Verification items for the finished model (mm, model axes). A direction names the side the tool comes from. Round coordinates to 2 decimals unless told otherwise and drop trailing zeros. Order: outer loops, then holes, each group sorted by start corner. A loop starts at its lowest first (then second) coordinate and runs counter-clockwise, first axis right, second up. Notation, with made-up numbers: (10, 69.5) -> (49, 69.5) arc R17 cw to (49, 96.5) -> close; hole circle Ø1 at (-19, -35). An arc over 180 degrees is marked (long way). Return JSON: item names as keys, results as strings. Group by question number.
Item 1: Draft check along Z on faces 4 (the flat face through (19, 63, 1)), 5 (the flat face through (10, 26, 7)), 6 (the flat face through (10.14, 18.43, 19.94)). Enter one of: pulls with the +Z half, pulls with the -Z half, needs draft (parallel to the pull), parting line crosses it, or undercut.
Item 2: Sectioned sample at B-B on x = 55. Record the cut outline in (y, z) (3 decimals), plus the area to 3 significant figures.
Item 3: Depth check by flat-ended pin: pin 1 Ø1.6 at (x, y) = (10.5, 8.5) entering from -Z; pin 2 Ø4.5 at (x, y) = (55, 53) entering from +Z; pin 3 Ø12 at (x, z) = (57, -40) entering from -Y; pin 4 Ø3 at (x, y) = (41.5, 45.5) entering from -Z. Enter the tip coordinate at first touch or a pass-through.
Item 4: Scan lines: probe 1 along Y at (x, z) = (13, -5.5); probe 2 along Y at (x, z) = (55, 46); probe 3 along Z at (x, y) = (26.5, 50) (3 decimals). Record each from-to range of solid material in increasing order. Write a range as from..to.
Item 5: Sectioned sample at C-C on z = -32. Record the cut outline in (x, y), plus the area to 3 significant figures.
Item 6: Sectioned sample at A-A on y = 53. Record the cut outline in (x, z) (3 decimals), plus the area to 3 significant figures.
Item 7: Access from +Z, -Z, +X, -X, +Y, -Y to the whole of each face (thin tool, end or side, straight path). Record for faces 1 (the flat face through (35, 53, 34.545)), 2 (the flat face through (45, 43, 42)), 3 (the flat face through (10, 6, -7)).
Item 8: Sectioned sample at D-D on y = 14.5. Record the cut outline in (x, z).
```python
from build123d import *

# Parameters (mm, degrees)
BOSS_EXTRUDE1_DEPTH = 20
CUT_EXTRUDE1_DEPTH  = 20
SKETCH4_W           = 15
SKETCH4_H           = 20
BOSS_EXTRUDE2_DEPTH = 50
SKETCH5_R           = 2.5
CUT_EXTRUDE2_DEPTH  = 137.703431193
SKETCH6_W           = 8
SKETCH6_H           = 15
CUT_EXTRUDE3_DEPTH  = 95.465374741
CUT_EXTRUDE4_DEPTH  = 95.465374741


with BuildPart() as part:
    # Sketch1 → Boss-Extrude1 (new body)
    with BuildSketch(Plane(origin=(0, 0, 0), x_dir=(0, 0, -1), z_dir=(1, 0, 0))):
        Polygon((15, 0), (-15, 0), (-49.545, 31.5), (-49.545, 63), (49.545, 63), (49.545, 31.5), align=None)
    extrude(amount=BOSS_EXTRUDE1_DEPTH)

    # Sketch3 → Cut-Extrude1 (cut)
    with BuildSketch(Plane(origin=(20, 0, 0), x_dir=(0, 0, -1), z_dir=(1, 0, 0))):
        Polygon((-10, 12.875), (-10, 6), (-3.125, 6), (-3.125, 8), (-4, 8), (-4, 10), (4, 10), (4, 8), (3.125, 8), (3.125, 6), (10, 6), (10, 12.875), (8, 12.875), (8, 12), (6, 12), (6, 20), (8, 20), (8, 19.125), (10, 19.125), (10, 26), (3.125, 26), (3.125, 24), (4, 24), (4, 22), (-4, 22), (-4, 24), (-3.125, 24), (-3.125, 26), (-10, 26), (-10, 19.125), (-8, 19.125), (-8, 20), (-6, 20), (-6, 12), (-8, 12), (-8, 12.875), align=None)
    extrude(amount=-CUT_EXTRUDE1_DEPTH, mode=Mode.SUBTRACT)

    # Sketch4 → Boss-Extrude2 (add)
    with BuildSketch(Plane(origin=(20, 0, 0), x_dir=(0, 0, -1), z_dir=(1, 0, 0))):
        with Locations((-42.045, 53)):
            Rectangle(SKETCH4_W, SKETCH4_H)
        with Locations((42.040757, 53)):
            Rectangle(SKETCH4_W, SKETCH4_H)
    extrude(amount=BOSS_EXTRUDE2_DEPTH)

    # Sketch5 → Cut-Extrude2 (cut, through all)
    with BuildSketch(Plane.XY.offset(49.545)):
        with Locations((55, 53)):
            Circle(SKETCH5_R)
    extrude(amount=-CUT_EXTRUDE2_DEPTH, mode=Mode.SUBTRACT)

    # Sketch6 → Cut-Extrude3 (cut, through all)
    with BuildSketch(Plane(origin=(20, 0, 0), x_dir=(0, 0, -1), z_dir=(1, 0, 0))):
        with Locations((-30.545, 53)):
            Rectangle(SKETCH6_W, SKETCH6_H)
        with Locations((30.540757, 53)):
            Rectangle(SKETCH6_W, SKETCH6_H)
    extrude(amount=-CUT_EXTRUDE3_DEPTH, mode=Mode.SUBTRACT)

    # Sketch7 → Cut-Extrude4 (cut, through all)
    with BuildSketch(Plane(origin=(20, 0, 0), x_dir=(0, 0, -1), z_dir=(1, 0, 0))):
        Polygon((-49.545, 43), (-24.740965738, 36.353779051), (-15, 0), (-52.774772494, 23.355056254), align=None)
        Polygon((49.540757, 43), (24.740965738, 36.353779051), (15, 0), (56.193227383, 18.176889525), align=None)
    extrude(amount=-CUT_EXTRUDE4_DEPTH, mode=Mode.SUBTRACT)


solid = part.part
```
Recorded:
{
 "1": {"face 4": "needs draft", "face 5": "undercut", "face 6": "pulls with the +Z half"},
 "2": {"outline": "(43, -49.541) -> (50.5, -49.541) -> (50.5, -34.541) -> (43, -34.541) -> close; (43, 34.545) -> (50.5, 34.545) -> (50.5, 49.545) -> (43, 49.545) -> close; (55.5, -49.541) -> (63, -49.541) -> (63, -34.541) -> (55.5, -34.541) -> close; (55.5, 34.545) -> (63, 34.545) -> (63, 49.545) -> (55.5, 49.545) -> close", "area": "450 mm²"},
 "3": {"pin 1": "z = -17.49", "pin 2": "through", "pin 3": "y = 43", "pin 4": "z = -49.54"},
 "4": {"probe 1": "0..6, 26..63", "probe 2": "43..50.5, 55.5..63", "probe 3": "-49.541..-34.541, 34.545..49.545"},
 "5": {"outline": "(0, 38.3) -> (20, 38.3) -> (20, 45.5) -> (0, 45.5) -> close; (0, 60.5) -> (20, 60.5) -> (20, 63) -> (0, 63) -> close", "area": "194 mm²"},
 "6": {"outline": "(0, -49.545) -> (20, -49.545) -> (20, -49.541) -> (52.5, -49.541) -> (52.5, -34.541) -> (0, -34.541) -> close; (0, -26.541) -> (20, -26.541) -> (20, 26.545) -> (0, 26.545) -> close; (0, 34.545) -> (52.5, 34.545) -> (52.5, 49.545) -> (0, 49.545) -> close; (57.5, -49.541) -> (70, -49.541) -> (70, -34.541) -> (57.5, -34.541) -> close; (57.5, 34.545) -> (70, 34.545) -> (70, 49.545) -> (57.5, 49.545) -> close", "area": "3,010 mm²"},
 "7": {"face 1": "+X", "face 2": "+Z, -Z, +X, -Y", "face 3": "+X, -X"},
 "8": {"outline": "(0, -18.89) -> (20, -18.89) -> (20, -6) -> (0, -6) -> close; (0, 6) -> (20, 6) -> (20, 18.89) -> (0, 18.89) -> close"}
}
